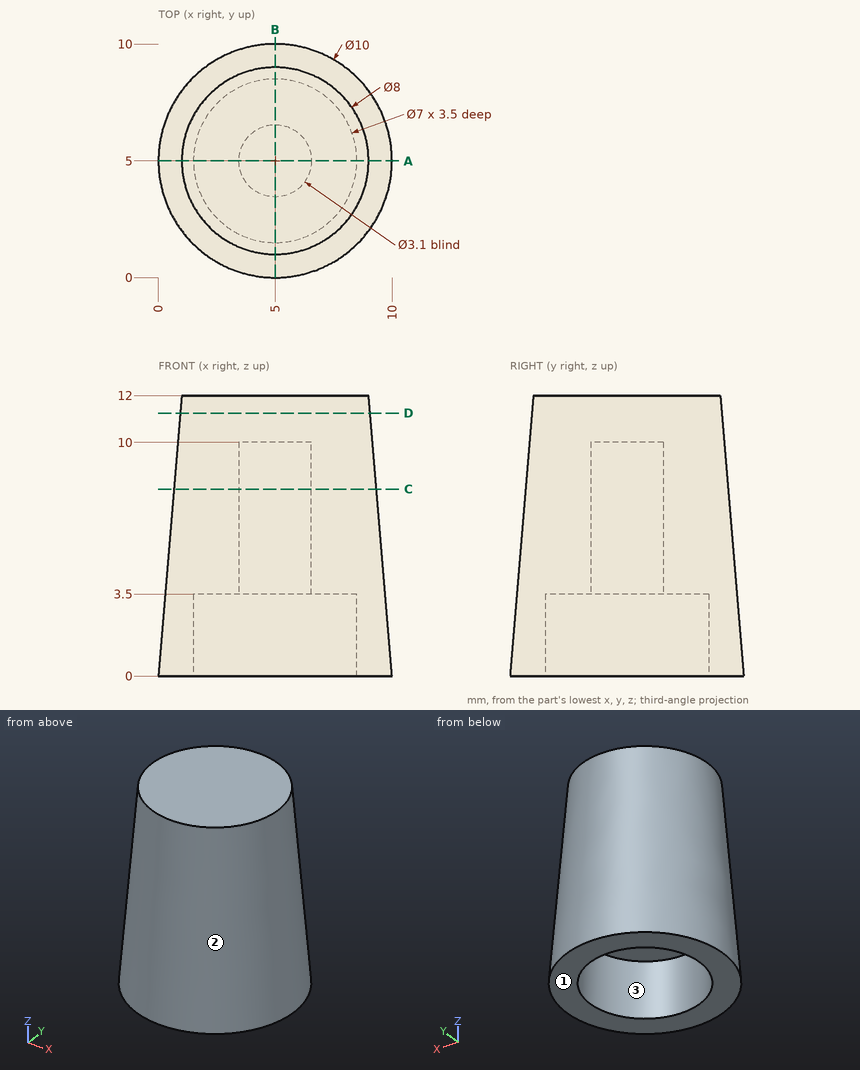
Design review of the part shown in the three views and the two pictorial views. Dimensions are in mm from the part's minimum x, y and z. Give positions to 0.01 mm unless a question says otherwise; leave off trailing zeros. Order: outer loops, then holes, each group sorted by start corner. A loop starts at its lowest first (then second) coordinate and runs counter-clockwise, first axis right, second up. Notation, with made-up numbers: (37, 65) -> (64, 65) arc R32 cw to (64, 92) -> close; hole circle Ø10 at (57, 14). An arc over 180 degrees is marked (long way). Write each question's results on one line, items separated by ' | '. Start each with the question number.
Q1. Add section D-D on z = 11.25. Give the boundary of the cut face in (x, y) (1 decimal), and give its area (3 significant figures).
Q2. Add section A-A on y = 5. Give the boundary of the cut face in (x, z), and give its area (4 significant figures).
Q3. Mouldability with a two-part tool opening along Y and no side actions: class the marked faces 1, 2 and 3 as +Y half, -Y half, draft (parallel to the pull), parting line (faces both ways), or undercut.
Q4. Add section C-C on z = 8. Give the boundary of the cut face in (x, y).
Q5. For pin 1 (2.5 mm diameter, centred on x = 5.5, y = 4.5, fed in from -Z); pin 2 (1 mm diameter, centred on x = 1.5, z = 6, fed in from +Y); pin 3 (3 mm diameter, centred on x = 6.5, z = 5, fed in from -Y), all flat-tipped, find the tip position at first contact; note any pin that passes through.
Q6. Wall thickness on L1, parallel to Z at x = 4, y = 4.25; L2, parallel to X at y = 4.5, z = 2.5; L3, parallel to Y at x = 5, z = 1.3: over which ranges is each line inside the solid? List them lowest first. Write a range as from..to.
Found:
1) outline: circle Ø8.1 at (5, 5) | area: 51.8 mm2
2) outline: (0, 0) -> (1.5, 0) -> (1.5, 3.5) -> (3.45, 3.5) -> (3.45, 10) -> (6.55, 10) -> (6.55, 3.5) -> (8.5, 3.5) -> (8.5, 0) -> (10, 0) -> (9, 12) -> (1, 12) -> close | area: 63.35 mm2
3) face 1: draft | face 2: parting line | face 3: undercut
4) outline: circle Ø8.67 at (5, 5); hole circle Ø3.1 at (5, 5)
5) pin 1: stops at z = 3.5 | pin 2: stops at y = 8.36 | pin 3: stops at y = 0.35
6) L1: z = 10..12 | L2: x = 0.23..1.54, 8.46..9.77 | L3: y = 0.11..1.5, 8.5..9.89
